Could you check a few things on this model? Use its own coordinates, in mm. Coordinates: 2 decimals unless noted, no trailing zeros. Write each loop counter-clockwise with the first axis right and the second up, starting at its lowest first coordinate (ties: lowest second). Pieces come first, ordered by that corner, then holes. Notation, with made-up numbers: (-5, 2.25) - (6, 2.25) arc R29 cw to (6, 23.25) - close; hole circle Ø7 at (-29.5, 10). An arc over 180 degrees is marked (long way). Answer as a JSON object with one key per item and string values. Group by question number.
1) If we section it at A-A (x = 0): State how many separate pieces and enclosed holes the cut face has, plus the area to 3 significant figures.
2) If we section it at C-C (z = 90.17): Write out the boundary of the cut face in (x, y).
3) Please list where these lines run through material, in increasing order: line 1 along X through (y, z) = (2, -54); line 2 along Z through (x, y) = (-12.7, 2.75) (3 decimals); line 3 along X through (y, z) = (5, 63).
4) If we section it at B-B (x = 12.7): Write out the boundary of the cut face in (y, z) (3 decimals), plus the area to 3 significant figures.
5) Will these pins go through, and if not, where does the flat tip stop? pin 1 Ø8 at (x, z) = (0, -73.025) entering from +Y; pin 2 Ø1.9 at (y, z) = (2.5, -69) entering from +X; pin 3 Ø2 at (y, z) = (2, 79.5) entering from -X; pin 4 Ø3 at (y, z) = (2, 58.5) entering from -X.
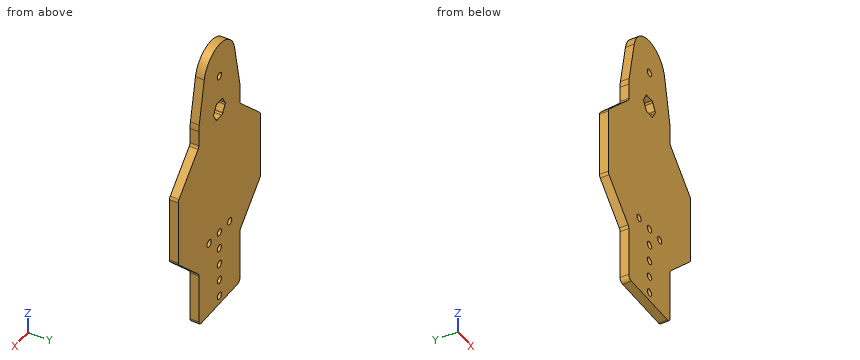
```python
from build123d import *

# Parameters (mm, degrees)
SKETCH1_R           = 2.5527
BOSS_EXTRUDE1_DEPTH = 6.35


with BuildPart() as part:
    # Sketch1 → Boss-Extrude1 (new body)
    with BuildSketch(Plane.XZ):
        with BuildLine():
            Line((-50.8, 24.084871939), (-50.8, -24.084871939))
            ThreePointArc((-50.8, -24.084871939), (-50.558317516, -25.299891837), (-49.87006403, -26.32993597))
            Line((-49.87006403, -26.32993597), (-26.32993597, -49.87006403))
            ThreePointArc((-26.32993597, -49.87006403), (-25.641682484, -50.900108163), (-25.4, -52.115128061))
            Line((-25.4, -52.115128061), (-25.4, -88.9))
            ThreePointArc((-25.4, -88.9), (-24.47006403, -91.14506403), (-22.225, -92.075))
            Line((-22.225, -92.075), (22.225, -92.075))
            ThreePointArc((22.225, -92.075), (24.47006403, -91.14506403), (25.4, -88.9))
            Line((25.4, -88.9), (25.4, -52.115128061))
            ThreePointArc((25.4, -52.115128061), (25.641682484, -50.900108163), (26.32993597, -49.87006403))
            Line((26.32993597, -49.87006403), (49.87006403, -26.32993597))
            ThreePointArc((49.87006403, -26.32993597), (50.558317516, -25.299891837), (50.8, -24.084871939))
            Line((50.8, -24.084871939), (50.8, 24.084871939))
            ThreePointArc((50.8, 24.084871939), (50.558317516, 25.299891837), (49.87006403, 26.32993597))
            Line((49.87006403, 26.32993597), (26.32993597, 49.87006403))
            ThreePointArc((26.32993597, 49.87006403), (25.641682484, 50.900108163), (25.4, 52.115128061))
            Line((25.4, 52.115128061), (25.4, 63.5))
            ThreePointArc((25.4, 63.5), (25.281197373, 65.953784703), (24.925900837, 68.384615385))
            Line((24.925900837, 68.384615385), (18.694425628, 100.183461538))
            ThreePointArc((18.694425628, 100.183461538), (0, 115.57), (-18.694425628, 100.183461538))
            Line((-18.694425628, 100.183461538), (-24.925900837, 68.384615385))
            ThreePointArc((-24.925900837, 68.384615385), (-25.281197373, 65.953784703), (-25.4, 63.5))
            Line((-25.4, 63.5), (-25.4, 52.115128061))
            ThreePointArc((-25.4, 52.115128061), (-25.641682484, 50.900108163), (-26.32993597, 49.87006403))
            Line((-26.32993597, 49.87006403), (-49.87006403, 26.32993597))
            ThreePointArc((-49.87006403, 26.32993597), (-50.558317516, 25.299891837), (-50.8, 24.084871939))
        make_face()
        with Locations((0, 90.17)):
            Circle(SKETCH1_R, mode=Mode.SUBTRACT)
        with Locations((0, -85.725)):
            Circle(SKETCH1_R, mode=Mode.SUBTRACT)
        with Locations((0, -73.025)):
            Circle(SKETCH1_R, mode=Mode.SUBTRACT)
        with Locations((0, -60.325)):
            Circle(SKETCH1_R, mode=Mode.SUBTRACT)
        with Locations((0, -47.625)):
            Circle(SKETCH1_R, mode=Mode.SUBTRACT)
        with Locations((0, -34.925)):
            Circle(SKETCH1_R, mode=Mode.SUBTRACT)
        with Locations((-12.7, -34.925)):
            Circle(SKETCH1_R, mode=Mode.SUBTRACT)
        with Locations((12.7, -34.925)):
            Circle(SKETCH1_R, mode=Mode.SUBTRACT)
        with BuildLine():
            Line((-6.872513185, 64.423457988), (-4.235994669, 68.990042012))
            ThreePointArc((-4.235994669, 68.990042012), (-4.173607217, 69.126443703), (-4.137993663, 69.272146448))
            ThreePointArc((-4.137993663, 69.272146448), (-3.702835951, 69.9135), (-2.929828627, 69.969680857))
            ThreePointArc((-2.929828627, 69.969680857), (-2.785839571, 69.927671726), (-2.636518516, 69.9135))
            Line((-2.636518516, 69.9135), (2.636518516, 69.9135))
            ThreePointArc((2.636518516, 69.9135), (2.785839571, 69.927671726), (2.929828627, 69.969680857))
            ThreePointArc((2.929828627, 69.969680857), (3.702835951, 69.9135), (4.137993663, 69.272146448))
            ThreePointArc((4.137993663, 69.272146448), (4.173607217, 69.126443703), (4.235994669, 68.990042012))
            Line((4.235994669, 68.990042012), (6.872513185, 64.423457988))
            ThreePointArc((6.872513185, 64.423457988), (6.959446788, 64.301228024), (7.06782229, 64.197534409))
            ThreePointArc((7.06782229, 64.197534409), (7.405671903, 63.5), (7.06782229, 62.802465591))
            ThreePointArc((7.06782229, 62.802465591), (6.959446788, 62.698771976), (6.872513185, 62.576542012))
            Line((6.872513185, 62.576542012), (4.235994669, 58.009957988))
            ThreePointArc((4.235994669, 58.009957988), (4.173607217, 57.873556297), (4.137993663, 57.727853552))
            ThreePointArc((4.137993663, 57.727853552), (3.702835951, 57.0865), (2.929828627, 57.030319143))
            ThreePointArc((2.929828627, 57.030319143), (2.785839571, 57.072328274), (2.636518516, 57.0865))
            Line((2.636518516, 57.0865), (-2.636518516, 57.0865))
            ThreePointArc((-2.636518516, 57.0865), (-2.785839571, 57.072328274), (-2.929828627, 57.030319143))
            ThreePointArc((-2.929828627, 57.030319143), (-3.702835951, 57.0865), (-4.137993663, 57.727853552))
            ThreePointArc((-4.137993663, 57.727853552), (-4.173607217, 57.873556297), (-4.235994669, 58.009957988))
            Line((-4.235994669, 58.009957988), (-6.872513185, 62.576542012))
            ThreePointArc((-6.872513185, 62.576542012), (-6.959446788, 62.698771976), (-7.06782229, 62.802465591))
            ThreePointArc((-7.06782229, 62.802465591), (-7.405671903, 63.5), (-7.06782229, 64.197534409))
            ThreePointArc((-7.06782229, 64.197534409), (-6.959446788, 64.301228024), (-6.872513185, 64.423457988))
        make_face(mode=Mode.SUBTRACT)
    extrude(amount=-BOSS_EXTRUDE1_DEPTH)


solid = part.part
```
Here are the results:
{
 "1": {"separate pieces": "8", "enclosed holes": "0", "area": "1,040 mm²"},
 "2": {"outline": "(-20.66, 0) - (-2.55, 0) - (-2.55, 6.35) - (-20.66, 6.35) - close; (2.55, 0) - (20.66, 0) - (20.66, 6.35) - (2.55, 6.35) - close"},
 "3": {"line 1": "x = -25.4 to 25.4", "line 2": "z = -92.075 to -37.478, -32.372 to 110.719", "line 3": "x = -25.4 to -7.25, 7.25 to 25.4"},
 "4": {"outline": "(0, -92.075) - (6.35, -92.075) - (6.35, -37.478) - (0, -37.478) - close; (0, -32.372) - (6.35, -32.372) - (6.35, 110.719) - (0, 110.719) - close", "area": "1,260 mm²"},
 "5": {"pin 1": "stops at y = 6.35", "pin 2": "stops at x = 25.4", "pin 3": "stops at x = -22.94", "pin 4": "stops at x = -25.4"}
}
